from build123d import *

# Parameters (mm, degrees)
SKETCH_1_W          = 27.5
SKETCH_1_H          = 27.5
EXTRUDE_1_DEPTH     = 1
SKETCH_2_R          = 1
CUT_EXTRUDE_1_DEPTH = 1
EXTRUDE_2_DEPTH     = 4
EXTRUDE_3_DEPTH     = 4.26
SKETCH_5_R          = 1.6
EXTRUDE_4_DEPTH     = 0.3
FILLET_1_R          = 0.5


with BuildPart() as part:
    # 草图1 → 凸台-拉伸1 (new body)
    with BuildSketch(Plane(origin=(0, 0, 0), x_dir=(1, 0, 0), z_dir=(0, 1, 0))):
        Rectangle(SKETCH_1_W, SKETCH_1_H)
    extrude(amount=EXTRUDE_1_DEPTH)

    # 草图2 → 切除-拉伸1 (cut)
    with BuildSketch(Plane(origin=(0, 1, 0), x_dir=(1, 0, 0), z_dir=(0, 1, 0))):
        with Locations(Location((-12.447971734, 12.492096903, 0), (0, 0, 270))):
            Circle(SKETCH_2_R)
        with Locations(Location((12.552028266, 12.492096903, 0), (0, 0, 270))):
            Circle(SKETCH_2_R)
        with Locations(Location((12.552028266, -12.507903097, 0), (0, 0, 270))):
            Circle(SKETCH_2_R)
        with Locations(Location((-12.447971734, -12.507903097, 0), (0, 0, 270))):
            Circle(SKETCH_2_R)
    extrude(amount=-CUT_EXTRUDE_1_DEPTH, mode=Mode.SUBTRACT)

    # 草图3 → 凸台-拉伸2 (add)
    with BuildSketch(Plane(origin=(0, 1, 0), x_dir=(1, 0, 0), z_dir=(0, 1, 0))):
        Polygon((-9.5, 12.05), (-12.1, 9.5), (-12.1, -9.5), (-9.5, -12.05), (9.5, -12.05), (12.1, -9.5), (12.1, 9.5), (9.5, 12.05), align=None)
    extrude(amount=EXTRUDE_2_DEPTH)

    # 草图4 → 凸台-拉伸3 (add)
    with BuildSketch(Plane.XZ):
        with BuildLine():
            Line((-9.5, 12.5), (9.5, 12.5))
            ThreePointArc((9.5, 12.5), (11.621320344, 11.621320344), (12.5, 9.5))
            Line((12.5, 9.5), (12.5, -9.5))
            ThreePointArc((12.5, -9.5), (11.621320344, -11.621320344), (9.5, -12.5))
            Line((9.5, -12.5), (-9.5, -12.5))
            ThreePointArc((-9.5, -12.5), (-11.621320344, -11.621320344), (-12.5, -9.5))
            Line((-12.5, -9.5), (-12.5, 9.5))
            ThreePointArc((-12.5, 9.5), (-11.621320344, 11.621320344), (-9.5, 12.5))
        make_face()
    extrude(amount=EXTRUDE_3_DEPTH)

    # 草图5 → 凸台-拉伸4 (add)
    with BuildSketch(Plane.XZ.offset(4.26)):
        with Locations(Location((2.5, 0.5, 0), (0, 0, 270))):
            Circle(SKETCH_5_R)
    extrude(amount=EXTRUDE_4_DEPTH)

    # 圆角1
    fillet_1_edges = [part.edges().sort_by_distance(p)[0] for p in [
        (-11.621320344, -4.26, 11.621320344),
        (-12.5, -4.26, 0),
        (-11.621320344, -4.26, -11.621320344),
        (0, -4.26, -12.5),
        (11.621320344, -4.26, -11.621320344),
        (12.5, -4.26, 0),
        (11.621320344, -4.26, 11.621320344),
        (0, -4.26, 12.5),
    ]]
    fillet(fillet_1_edges, radius=FILLET_1_R)


solid = part.part
Read the model definition and answer for the solid it produces. Units are mm, in the model's axes. A direction names the side the tool comes from. Round coordinates to 2 decimals unless told otherwise and drop trailing zeros. Write each loop counter-clockwise with the first axis right and the second up, starting at its lowest first coordinate (ties: lowest second). Pieces come first, ordered by that corner, then holes. Notation, with made-up numbers: M -24,22 L -15,22 A24 ccw -15,56 Z; hole C -22,20 d1. An arc over 180 degrees is marked long. Use a Markdown table: item, result.
1) The part is cut by section B-B (z = 0.5). Write down the section's boundary in (x, y), plus the area to 3 significant figures.
Answers follow:
| item | result |
|---|---|
| outline | M -13.75,0 L -12.5,0 L -12.5,-3.76 A0.5 ccw -12,-4.26 L 0.9,-4.26 L 0.9,-4.56 L 4.1,-4.56 L 4.1,-4.26 L 12,-4.26 A0.5 ccw 12.5,-3.76 L 12.5,0 L 13.75,0 L 13.75,1 L 12.1,1 L 12.1,5 L -12.1,5 L -12.1,1 L -13.75,1 Z |
| area | 232 mm2 |
2) The part is cut by section D-D (x = 2.5). Write down the section's boundary in (y, z).
Answers follow:
| item | result |
|---|---|
| outline | M -4.56,-1.1 L -4.26,-1.1 L -4.26,-12 A0.5 ccw -3.76,-12.5 L 0,-12.5 L 0,-13.75 L 1,-13.75 L 1,-12.05 L 5,-12.05 L 5,12.05 L 1,12.05 L 1,13.75 L 0,13.75 L 0,12.5 L -3.76,12.5 A0.5 ccw -4.26,12 L -4.26,2.1 L -4.56,2.1 Z |
3) Flat-ended cylindrical pins translate along their axes: pin 1 (1.2 mm diameter, centred on x = 3.5, y = 2, fed in from -Z); pin 2 (1.9 mm diameter, centred on x = 0, y = -2.5, fed in from +Z); pin 3 (4 mm diameter, centred on x = -9, z = -10, fed in from -Y). Find the tip coordinate at first contact, or state that the pin passes through.
Answers follow:
| item | result |
|---|---|
| pin 1 | stops at z = -12.05 |
| pin 2 | stops at z = 12.5 |
| pin 3 | stops at y = -4.26 |
4) For a pull along X with two mould halves and no side action, classify faces 6 (the flat face through (13.75, 0.5, 0.2)), 7 (the flat face through (-12.5, -2, 0)), 8 (the flat face through (3, -4.56, 1)), 9 (the cylindrical face through (-11.605, 0.507, 13.045)) as pulls with the +X half, pulls with the -X half, needs draft (parallel to the pull), parting line crosses it, or undercut.
Answers follow:
| item | result |
|---|---|
| face 6 | pulls with the +X half |
| face 7 | pulls with the -X half |
| face 8 | needs draft |
| face 9 | undercut |
5) A tool of negligible diameter and unlimited length cuts with its end or side. For faces 1 (the cylindrical face through (-11.64, -1.85, 11.6)), 2 (the flat face through (0, -2, -12.5)), 3 (the flat face through (-12.1, 3, 0)), 4 (the flat face through (12.1, 3, 0)), 5 (the flat face through (-10.782, 2.972, -10.793)), from which of +Z, -Z, +X, -X, +Y, -Y can it reach the whole face along a straight path? Write none if from no direction.
Answers follow:
| item | result |
|---|---|
| face 1 | +Z, -X, -Y |
| face 2 | -Z, +X, -X, -Y |
| face 3 | +Z, -Z, -X, +Y |
| face 4 | +Z, -Z, +X, +Y |
| face 5 | -Z, -X, +Y |
6) Straight lines are drawn through the part: line 1 along Z through (x, y) = (-3.75, -3.5); line 2 along X through (y, z) = (4, -7.75). For each, find the intervals that lie inside material, in ascending order. Write a range as [from, to].
Answers follow:
| item | result |
|---|---|
| line 1 | z = [-12.5, 12.5] |
| line 2 | x = [-12.1, 12.1] |
7) The part is cut by section C-C (y = 1.5). Write down the section's boundary in (x, z).
Answers follow:
| item | result |
|---|---|
| outline | M -12.1,-9.5 L -9.5,-12.05 L 9.5,-12.05 L 12.1,-9.5 L 12.1,9.5 L 9.5,12.05 L -9.5,12.05 L -12.1,9.5 Z |
8) The part is cut by section A-A (x = -5.75). Write down the section's boundary in (y, z).
Answers follow:
| item | result |
|---|---|
| outline | M -4.26,-12 A0.5 ccw -3.76,-12.5 L 0,-12.5 L 0,-13.75 L 1,-13.75 L 1,-12.05 L 5,-12.05 L 5,12.05 L 1,12.05 L 1,13.75 L 0,13.75 L 0,12.5 L -3.76,12.5 A0.5 ccw -4.26,12 Z |
